Input: part model. Units: mm. Frame: model coordinates. Face numbers are marked on the shaded views. Coordinates: 2 decimals unless noted, no trailing zeros. Order: outer loops, then holes, each group sorted by start corner. A loop starts at its lowest first (then second) coordinate and runs counter-clockwise, first axis right, second up. Notation, with made-up numbers: (74, -37.75) -> (107, -37.75) arc R26 ccw to (107, -23.75) -> close; hole circle Ø3 at (70.25, 18.5). An arc over 180 degrees is marked (long way). Answer as CSV lines item,"result".
from build123d import *

# Parameters (mm, degrees)
F0_R     = 45
F1_DEPTH = 20
F2_T     = -2
F3_R     = 12
F4_DEPTH = 18
F5_T     = -2
F7_DEPTH = 18
F8_R     = 1


# Not quite as in the source:
# - a shell that OpenCascade refuses in one call is made with other operations: the cavity is built on its own and cut out


with BuildPart() as f1:
    # F0 (on Top) → F1 (new body)
    with BuildSketch(Plane.XY):
        Circle(F0_R)
    extrude(amount=F1_DEPTH)

    # F2
    f2_openings = [f1.faces().sort_by_distance(p)[0] for p in [
        (0, 0, 0),
    ]]
    offset(amount=F2_T, openings=f2_openings)

    # F3 (on Top) → F4 (join, through all)
    with BuildSketch(Plane.XY):
        Circle(F3_R)
    extrude(amount=F4_DEPTH)

    # F5: a shell. OpenCascade refuses it in one call, so the cavity is built on its own and cut out:
    # the body offset inwards by the wall thickness, plus a prism from it out through each open face.
    f5_core = offset(f1.part, amount=F5_T, kind=Kind.INTERSECTION, mode=Mode.PRIVATE)
    f5_exits = [f5_core.faces().sort_by_distance(p)[0] for p in [
        (0, 0, 2),
    ]]
    add(f5_core, mode=Mode.SUBTRACT)
    extrude(f5_exits, amount=-F5_T, mode=Mode.SUBTRACT)

    # F6 (on face) → F7 (cut, through all)
    with BuildSketch(Plane(origin=(0, 0, 0), x_dir=(1, 0, 0), z_dir=(0, 0, -1))):
        with BuildLine():
            ThreePointArc((10, 0), (9.9202969627, -1.2600429248), (9.6824583655, -2.5))
            Line((9.6824583655, -2.5), (11.7366945943, -2.5))
            ThreePointArc((11.7366945943, -2.5), (11.9339921052, -1.2569138531), (12, 0))
            ThreePointArc((12, 0), (11.9339921052, 1.2569138531), (11.7366945943, 2.5))
            Line((11.7366945943, 2.5), (9.6824583655, 2.5))
            ThreePointArc((9.6824583655, 2.5), (9.9202969627, 1.2600429248), (10, 0))
        make_face()
    extrude(amount=-F7_DEPTH, mode=Mode.SUBTRACT)

    # F8
    f8_edges = [f1.edges().sort_by_distance(p)[0] for p in [
        (-45, 0, 20),
    ]]
    fillet(f8_edges, radius=F8_R)


solid = f1.part
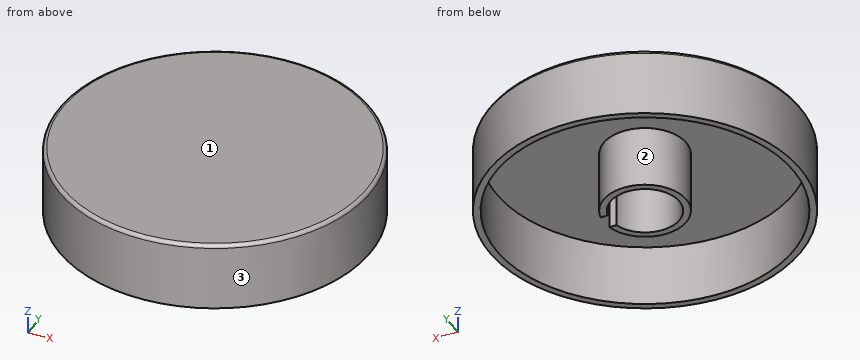
1. Cut plane B-B (y = 0). Return the cut outline in (x, z).
Findings:
outline,"(-45, 0) -> (-43, 0) -> (-43, 18) -> (-12, 18) -> (-12, 0) -> (-10, 0) -> (-10, 18) -> (43, 18) -> (43, 0) -> (45, 0) -> (45, 19) arc R1 ccw to (44, 20) -> (-44, 20) arc R1 ccw to (-45, 19) -> close"
2. Cut plane A-A (z = 13.5). Return the cut outline in (x, y).
Findings:
outline,"circle Ø90 at (0, 0); (9.68, -2.5) arc R10 cw (long way) to (9.68, 2.5) -> (11.74, 2.5) arc R12 ccw (long way) to (11.74, -2.5) -> close; hole circle Ø86 at (0, 0)"
3. Cut plane C-C (x = 0). Return the cut outline in (y, z), plus the area to 3 significant figures.
Findings:
outline,"(-45, 0) -> (-43, 0) -> (-43, 18) -> (-12, 18) -> (-12, 0) -> (-10, 0) -> (-10, 18) -> (10, 18) -> (10, 0) -> (12, 0) -> (12, 18) -> (43, 18) -> (43, 0) -> (45, 0) -> (45, 19) arc R1 ccw to (44, 20) -> (-44, 20) arc R1 ccw to (-45, 19) -> close"
area,"324 mm2"
4. Mould query, pull axis X, two halves, no side actions, for the marked faces 1, 2 and 3. Classes: released by +X, released by -X, zero draft, split by the parting line, or undercut.
Findings:
face 1,"zero draft"
face 2,"undercut"
face 3,"split by the parting line"
5. Contact query for flat-ended pins moving along their axis: pin 1 (1 mm diameter, centred on y = 34, z = 6, fed in from -X); pin 2 (8 mm diameter, centred on y = -18, z = 14, fed in from -X); pin 3 (2 mm diameter, centred on x = 22, y = 11.5, fed in from -Z). Output: stop coordinate, or through.
Findings:
pin 1,"stops at x = -30.05"
pin 2,"stops at x = -42.77"
pin 3,"stops at z = 18"
6. Ray query, line 1 along Y through (x, z) = (0, 5.25); line 2 along X through (y, z) = (2, 2); line 3 along Z through (x, y) = (36.5, -15.5). Return the intervals inside material, ascending.
Findings:
line 1,"y = -45 to -43, -12 to -10, 10 to 12, 43 to 45"
line 2,"x = -44.96 to -42.95, -11.83 to -9.8, 42.95 to 44.96"
line 3,"z = 18 to 20"
